Design review of the part shown in the three views and the two pictorial views. Dimensions are in mm from the part's minimum x, y and z. Coordinates: 2 decimals unless noted, no trailing zeros. Write each loop counter-clockwise with the first axis right and the second up, starting at its lowest first coordinate (ties: lowest second). Pieces come first, ordered by that corner, then holes. Notation, with made-up numbers: (-30.5, -13) -> (14.5, -13) arc R14 ccw to (14.5, 1) -> close; hole circle Ø7 at (23, -0.75). An arc over 180 degrees is marked (long way). Answer in a Markdown table with one row per item. Add a question column.
Item 1: To check wall thickness, follow line 1 (Y direction, x = 9.5, z = 14); line 2 (Z direction, x = 5.75, y = 2.75); line 3 (X direction, y = 9.5, z = 17). State the ranges of each line that lie inside material, in increasing order.
Item 2: Clearance check with flat-ended pins moving along their axes: P1, Ø6, axis at x = 13, z = 4, coming from the +Y side; P2, Ø1, axis at x = 4, z = 20.5, coming from the -Y side (1 decimal); P3, Ø3, axis at x = 6, z = 5, coming from the +Y side (1 decimal); P4, Ø3, axis at y = 19, z = 15.5, coming from the +X side. State where each tip first meets the part, or that it passes through.
Item 3: Draft analysis for pull direction Y (two halves, no side actions). For the marked faces 1, 2 and 3, state which applies: released by +Y, released by -Y, zero draft, split by the parting line, or undercut.
Item 4: Take a section at A-A, the plane z = 5.5. Write out the cut boundary in (x, y) (1 decimal).
Item 5: Take a section at B-B, the plane z = 13.5. Write out the cut boundary in (x, y).
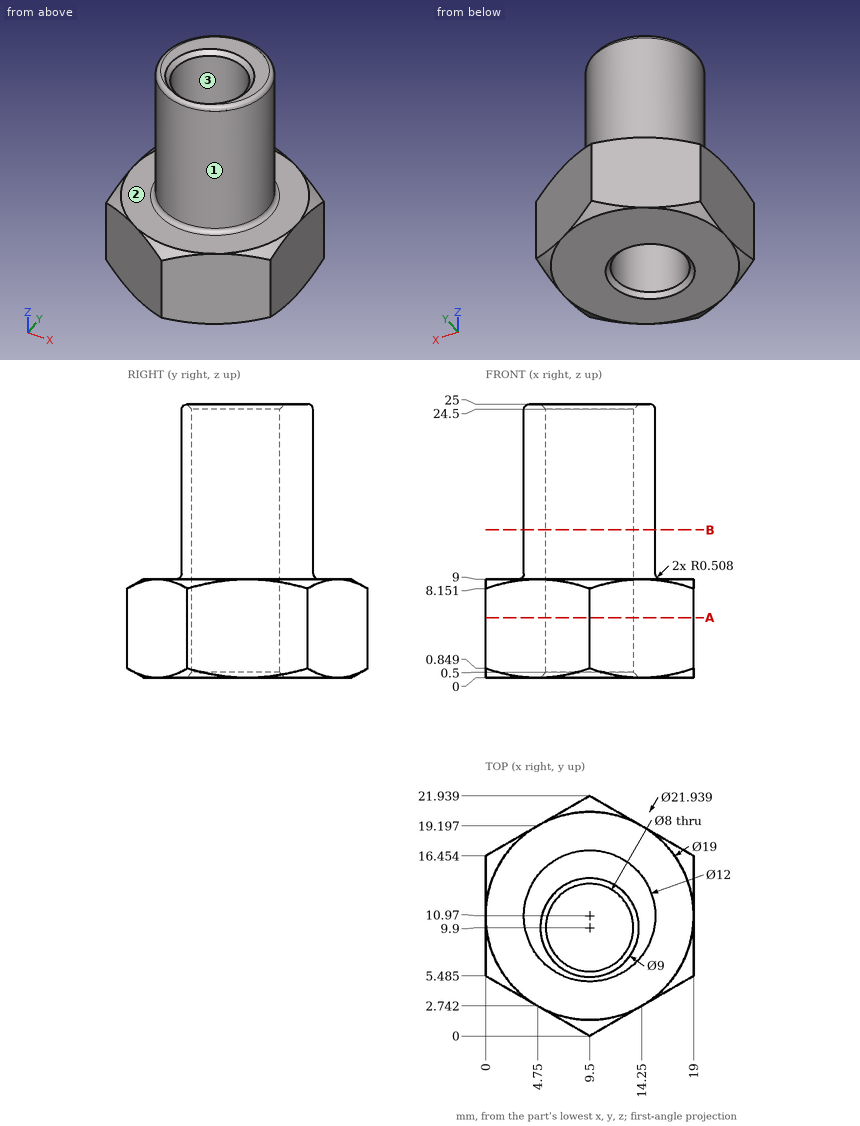
Answers:
| question | item | result |
|---|---|---|
| 1 | line 1 | y = 4.97 to 5.9, 13.9 to 16.97 |
| 1 | line 2 | z = 0 to 9 |
| 1 | line 3 | x = 3.68 to 5.52, 13.48 to 15.32 |
| 2 | P1 | stops at y = 21.65 |
| 2 | P2 | stops at y = 7.7 |
| 2 | P3 | stops at y = 20.8 |
| 2 | P4 | passes through |
| 3 | face 1 | split by the parting line |
| 3 | face 2 | zero draft |
| 3 | face 3 | undercut |
| 4 | outline | (0, 5.5) -> (9.5, 0) -> (19, 5.5) -> (19, 16.5) -> (9.5, 21.9) -> (0, 16.5) -> close; hole circle Ø8 at (9.5, 9.9) |
| 5 | outline | circle Ø12 at (9.5, 10.97); hole circle Ø8 at (9.5, 9.9) |
